Work out the finished part from the listing and answer in its coordinate system (mm). Round coordinates to 2 decimals unless told otherwise and drop trailing zeros. Write each loop counter-clockwise with the first axis right and the second up, starting at its lowest first coordinate (ties: lowest second). Pieces come first, ordered by that corner, then holes. Notation, with made-up numbers: (44, -5.75) -> (52, -5.75) arc R9 cw to (52, 3.25) -> close; hole circle Ø10 at (-11.75, 7). An arc over 180 degrees is marked (long way). Answer as a JSON object with one key per item and string values. Group by question number.
Autodesk Fusion 360 part; units mm, degrees
sketch "Sketch1" plane through (0, 0, 0) normal (0, 0, 1) x (1, 0, 0)
  line L0 (-20.19, -5) -> (0, -5)
  line L1 (0, -5) -> (0, 5)
  line L2 (0, 5) -> (-20.19, 5)
  line L3 (-20.19, 5) -> (-20.19, -5)
  line L4 (0, 5) -> (1, 5)
  line L5 (5, 1) -> (5, -1)
  line L6 (1, -5) -> (0, -5)
  line L7 (0, -5) -> (0, 5)
  arc A0 (1, -5) -> (5, -1) centre (1, -1) ccw
  arc A1 (5, 1) -> (1, 5) centre (1, 1) ccw
  circle A2 centre (0, 0) radius 2
  point P0 (5, 5)
  dimension "d1" = 20.19
  dimension "d2" = 10
  dimension "d3" = 5
  dimension "d5" = 4
  dimension "d6" = 4
  dimension "d7" = 4
extrude "Extrude1" add sketch "Sketch1" along normal mid plane 1 contours L0 L1 L2 L3 L7 A2 | L1 L4 L5 L6 L7 A0 A1 A2
chamfer "Chamfer1" distance 0.1 angle 45 2 edges at (-1.8647, 0.7232, 0.5) (-1.8647, -0.7232, -0.5)
1) Straight lines are drawn through the part: L1, parallel to X at y = 0, z = 0; L2, parallel to Y at x = 0, z = -0.1; L3, parallel to X at y = 1.25, z = -0.3. For each, find the intervals that lie inside material, in ascending order.
2) A cutting plane is placed at D-D on y = 3.25. Determine the outline of the cut face in (x, z), plus the area to 3 significant figures.
3) For a pull along X with two mould halves and no side action, classify faces 1 (the face through (5, 0, 0)), 2 (the face through (-20.19, 0, 0)), 3 (the face through (0, -2, 0)) as released by +X, released by -X, zero draft, split by the parting line, or undercut.
4) A cutting plane is placed at C-C on z = 0. Determine the outline of the cut face in (x, y), plus the area to 3 significant figures.
5) A cutting plane is placed at B-B on x = 0. Determine the outline of the cut face in (y, z), plus the area to 3 significant figures.
6) A cutting plane is placed at A-A on y = 0. Determine the outline of the cut face in (x, z), plus the area to 3 significant figures.
Established:
{
 "1": {"L1": "x = -20.19 to -2, 2 to 5", "L2": "y = -5 to -2, 2 to 5", "L3": "x = -20.19 to -1.56, 1.56 to 4.99"},
 "2": {"outline": "(-20.19, -0.5) -> (4.31, -0.5) -> (4.31, 0.5) -> (-20.19, 0.5) -> close", "area": "24.5 mm²"},
 "3": {"face 1": "released by +X", "face 2": "released by -X", "face 3": "undercut"},
 "4": {"outline": "(-20.19, -5) -> (1, -5) arc R4 ccw to (5, -1) -> (5, 1) arc R4 ccw to (1, 5) -> (-20.19, 5) -> close; hole circle Ø4 at (0, 0)", "area": "232 mm²"},
 "5": {"outline": "(-5, -0.5) -> (-2.1, -0.5) -> (-2, -0.4) -> (-2, 0.4) -> (-2.1, 0.5) -> (-5, 0.5) -> close; (2, -0.4) -> (2.1, -0.5) -> (5, -0.5) -> (5, 0.5) -> (2.1, 0.5) -> (2, 0.4) -> close", "area": "5.98 mm²"},
 "6": {"outline": "(-20.19, -0.5) -> (-2.1, -0.5) -> (-2, -0.4) -> (-2, 0.4) -> (-2.1, 0.5) -> (-20.19, 0.5) -> close; (2, -0.4) -> (2.1, -0.5) -> (5, -0.5) -> (5, 0.5) -> (2.1, 0.5) -> (2, 0.4) -> close", "area": "21.2 mm²"}
}
